from build123d import *

# Parameters (mm, degrees)
F0_R     = 19.05
F1_DEPTH = 3.175
F2_W     = 22.86
F2_H     = 11.938
F2_R     = 0.889
F3_DEPTH = 3.176
F5_DEPTH = 1.524


with BuildPart() as f1:
    # F0 (on Top) → F1 (new body)
    with BuildSketch(Plane.XY):
        Circle(F0_R)
    extrude(amount=F1_DEPTH)

    # F2 (on face) → F3 (cut, through all)
    with BuildSketch(Plane.XY.offset(3.175)):
        Rectangle(F2_W, F2_H)
        with Locations((-13.843, 0)):
            Circle(F2_R)
        with Locations((13.843, 0)):
            Circle(F2_R)
    extrude(amount=-F3_DEPTH, mode=Mode.SUBTRACT)

    # F4 (on face) → F5 (cut)
    with BuildSketch(Plane.XY.offset(3.175)):
        with BuildLine():
            Line((13.843, 2.6035), (-13.843, 2.6035))
            ThreePointArc((-13.843, 2.6035), (-16.4465, 0), (-13.843, -2.6035))
            Line((-13.843, -2.6035), (13.843, -2.6035))
            ThreePointArc((13.843, -2.6035), (16.4465, 0), (13.843, 2.6035))
        make_face()
    extrude(amount=-F5_DEPTH, mode=Mode.SUBTRACT)


solid = f1.part
Input: part model. Units: mm. Frame: model coordinates. A direction names the side the tool comes from. Give positions to 0.01 mm unless a question says otherwise; leave off trailing zeros. Loops run counter-clockwise (first coordinate to the right, second up) from the corner with the lowest first, then second, coordinate; pieces in that order, holes last. Notation, with made-up numbers: (42.25, 76) - (84.25, 76) arc R25 cw to (84.25, 110) - close; hole circle Ø1 at (62.5, -35.5). An arc over 180 degrees is marked (long way). Use CSV: the item, a comma, the result in double quotes. Start each with the question number.
Item 1: Section A-A on x = 0. Return loops of the section in (y, z) (3 decimals).
Item 2: Reachability of faces 4 (the flat face through (-13, -1, 1.651)), 5 (the flat face through (0, -8, 0)), 6 (the flat face through (11.43, 0, 1)) from +Z, -Z, +X, -X, +Y, -Y: full face, straight path, thin tool, end or side. Return the list, or none.
Item 3: Section B-B on y = 0. State how many separate pieces and enclosed holes the cut face has, then the cut area to 3 significant figures.
Item 4: Section D-D on x = 7. Return loops of the section in (y, z) (3 decimals), then the cut area to 3 significant figures.
Item 5: Section C-C on z = 0.95. Return loops of the section in (x, y).
Item 6: Mould query, pull axis Y, two halves, no side actions, for faces 1 (the flat face through (0, -8, 3.175)), 2 (the cylindrical face through (-15.12, -11.59, 1.57)), 3 (the cylindrical face through (-16.446, 0.057, 2.424)). Classes: pulls with the +Y half, pulls with the -Y half, needs draft (parallel to the pull), parting line crosses it, or undercut.
Item 7: Line query: line 1 (Y direction, x = 0, z = 0.3); line 2 (Y direction, x = 14, z = 2.3); line 3 (X direction, y = 1, z = 2.85). Output: solid intervals per line, ascending.
Item 8: Contact query for flat-ended pins moving along their axis: P1, Ø1.2, axis at x = -13, z = 3, coming from the +Y side; P2, Ø1.7, axis at x = 12.5, z = 2.5, coming from the -Y side; P3, Ø1.7, axis at x = 12.5, z = 2.5, coming from the +Y side; P4, Ø1.1, axis at x = -13.843, y = 0, coming from the +Z side. Output: stop coordinate, or through.
Ans:
1,outline,"(-19.05, 0) - (-5.969, 0) - (-5.969, 3.175) - (-19.05, 3.175) - close; (5.969, 0) - (19.05, 0) - (19.05, 3.175) - (5.969, 3.175) - close"
2,face 4,"+Z"
2,face 5,"-Z, +X, -X, +Y, -Y"
2,face 6,"+Z, -Z"
3,separate pieces,"4"
3,enclosed holes,"0"
3,area,"27.2 mm2"
4,outline,"(-17.717, 0) - (-5.969, 0) - (-5.969, 3.175) - (-17.717, 3.175) - close; (5.969, 0) - (17.717, 0) - (17.717, 3.175) - (5.969, 3.175) - close"
4,area,"74.6 mm2"
5,outline,"circle Ø38.1 at (0, 0); hole circle Ø1.78 at (-13.84, 0); hole (-11.43, -5.97) - (11.43, -5.97) - (11.43, 5.97) - (-11.43, 5.97) - close; hole circle Ø1.78 at (13.84, 0)"
6,face 1,"needs draft"
6,face 2,"parting line crosses it"
6,face 3,"undercut"
7,line 1,"y = -19.05 to -5.97, 5.97 to 19.05"
7,line 2,"y = -12.92 to -2.6, 2.6 to 12.92"
7,line 3,"x = -19.02 to -16.25, 16.25 to 19.02"
8,P1,"stops at y = 14.46"
8,P2,"stops at y = -15.07"
8,P3,"stops at y = 15.07"
8,P4,"passes through"
